Could you check a few things on this model? Use its own coordinates, in mm. A direction names the side the tool comes from. Give positions to 0.01 mm unless a question says otherwise; leave off trailing zeros. Order: outer loops, then holes, each group sorted by start corner. A loop starts at its lowest first (then second) coordinate and runs counter-clockwise, first axis right, second up. Notation, with made-up numbers: (-1.75, 44) -> (23.25, 44) arc R22 cw to (23.25, 60) -> close; hole circle Ø5 at (71.25, -21). An arc over 180 degrees is marked (long way). Use one line per item in the form item = value. Start each with the question number.
from build123d import *

# Parameters (mm, degrees)
BOSS_EXTRUDE13_OUTLINE_W = 40
BOSS_EXTRUDE13_OUTLINE_H = 40
BOSS_EXTRUDE13_OUTLINE_R = 2.5
BOSS_EXTRUDE13_DEPTH     = 5
SKETCH3_R                = 12
BOSS_EXTRUDE17_DEPTH     = 30
FILLET2_R                = 1
FILLET3_R                = 5
FILLET4_R                = 1
SKETCH6_R                = 16
BOSS_EXTRUDE18_DEPTH     = 6
SKETCH5_R                = 6.5
CUT_EXTRUDE2_DEPTH       = 55


# Read off the part's stored shape, not the designer's step: Boss-Extrude13
with BuildPart() as part:
    # Boss-Extrude13 outline → Boss-Extrude13 (new body)
    with BuildSketch(Plane(origin=(0, 0, 0), x_dir=(1, 0, 0), z_dir=(0, 1, 0))):
        Rectangle(BOSS_EXTRUDE13_OUTLINE_W, BOSS_EXTRUDE13_OUTLINE_H)
        with Locations((-15, -15.102802021)):
            Circle(BOSS_EXTRUDE13_OUTLINE_R, mode=Mode.SUBTRACT)
        with Locations((15.102802021, -15.102802021)):
            Circle(BOSS_EXTRUDE13_OUTLINE_R, mode=Mode.SUBTRACT)
        with Locations((-15, 15)):
            Circle(BOSS_EXTRUDE13_OUTLINE_R, mode=Mode.SUBTRACT)
        with Locations((15.102802021, 15)):
            Circle(BOSS_EXTRUDE13_OUTLINE_R, mode=Mode.SUBTRACT)
    extrude(amount=BOSS_EXTRUDE13_DEPTH)

    # Sketch3 → Boss-Extrude17 (add)
    with BuildSketch(Plane(origin=(0, 5, 0), x_dir=(1, 0, 0), z_dir=(0, 1, 0))):
        with Locations(Location((0, 0, 0), (0, 0, 270))):
            Circle(SKETCH3_R)
    extrude(amount=BOSS_EXTRUDE17_DEPTH)

    # Fillet2
    fillet2_edges = [part.edges().sort_by_distance(p)[0] for p in [
        (20, 5, 0),
        (0, 5, -20),
        (-20, 5, 0),
        (0, 5, 20),
    ]]
    fillet(fillet2_edges, radius=FILLET2_R)

    # Fillet3
    # the kernel refuses this fillet: 5 mm, written as the material it adds along each edge
    with BuildSketch(Plane(origin=(0, 5, 0), x_dir=(0, 0, 1), z_dir=(-1, 0, 0))) as fillet3_piece_1:
        with BuildLine():
            CenterArc((12 + FILLET3_R, FILLET3_R), FILLET3_R, 180, 90)
            Line((12, FILLET3_R), (12, 0))
            Line((12, 0), (12 + FILLET3_R, 0))
        make_face()
    revolve(axis=Axis((0, 5, 0), (0, 1, 0)))
    # the kernel refuses this fillet: 5 mm, written as the material it takes off along each edge
    with BuildSketch(Plane(origin=(-15, 5, -15), x_dir=(0, 0, -1), z_dir=(1, 0, 0))) as fillet3_2_piece_1:
        with BuildLine():
            CenterArc((4, -1), 1, 0, 90)
            Line((5, -1), (5, 0))
            Line((5, 0), (4, 0))
        make_face()
    revolve(axis=Axis((-15, 5, -15), (0, 1, 0)), revolution_arc=90, mode=Mode.SUBTRACT)
    with BuildSketch(Plane(origin=(15, 5, -15), x_dir=(1, 0, 0), z_dir=(0, 0, 1))) as fillet3_2_piece_2:
        with BuildLine():
            CenterArc((4, -1), 1, 0, 90)
            Line((5, -1), (5, 0))
            Line((5, 0), (4, 0))
        make_face()
    revolve(axis=Axis((15, 5, -15), (0, 1, 0)), revolution_arc=90, mode=Mode.SUBTRACT)
    with BuildSketch(Plane(origin=(-15, 5, 15), x_dir=(-1, 0, 0), z_dir=(0, 0, -1))) as fillet3_2_piece_3:
        with BuildLine():
            CenterArc((4, -1), 1, 0, 90)
            Line((5, -1), (5, 0))
            Line((5, 0), (4, 0))
        make_face()
    revolve(axis=Axis((-15, 5, 15), (0, 1, 0)), revolution_arc=90, mode=Mode.SUBTRACT)
    with BuildSketch(Plane(origin=(15, 5, 15), x_dir=(0, 0, 1), z_dir=(-1, 0, 0))) as fillet3_2_piece_4:
        with BuildLine():
            CenterArc((4, -1), 1, 0, 90)
            Line((5, -1), (5, 0))
            Line((5, 0), (4, 0))
        make_face()
    revolve(axis=Axis((15, 5, 15), (0, 1, 0)), revolution_arc=90, mode=Mode.SUBTRACT)
    with BuildSketch(Plane(origin=(20, -12.5, 20), x_dir=(-1, 0, 0), z_dir=(0, 1, 0)), Plane(origin=(20, -12.5, -20), x_dir=(0, 0, 1), z_dir=(0, 1, 0))) as fillet3_2_piece_5:
        with BuildLine():
            CenterArc((FILLET3_R, -FILLET3_R), FILLET3_R, 90, 90)
            Line((0, -FILLET3_R), (0, 0))
            Line((0, 0), (FILLET3_R, 0))
        make_face()
    extrude(amount=17.5, mode=Mode.SUBTRACT)
    with BuildSketch(Plane(origin=(-20, -12.5, 20), x_dir=(1, 0, 0), z_dir=(0, 1, 0)), Plane(origin=(-20, -12.5, -20), x_dir=(0, 0, 1), z_dir=(0, 1, 0))) as fillet3_2_piece_6:
        with BuildLine():
            CenterArc((FILLET3_R, FILLET3_R), FILLET3_R, 180, 90)
            Line((0, FILLET3_R), (0, 0))
            Line((0, 0), (FILLET3_R, 0))
        make_face()
    extrude(amount=17.5, mode=Mode.SUBTRACT)

    # Fillet4
    fillet4_edges = [part.edges().sort_by_distance(p)[0] for p in [
        (0, 35, -12),
    ]]
    fillet(fillet4_edges, radius=FILLET4_R)

    # Sketch6 → Boss-Extrude18 (add)
    with BuildSketch(Plane.XZ):
        with Locations(Location((0, 0, 0), (0, 0, 90))):
            Circle(SKETCH6_R)
    extrude(amount=BOSS_EXTRUDE18_DEPTH)

    # Sketch5 → Cut-Extrude2 (cut)
    with BuildSketch(Plane(origin=(0, 35, 0), x_dir=(1, 0, 0), z_dir=(0, 1, 0))):
        with Locations(Location((0, 0, 0), (0, 0, 270))):
            Circle(SKETCH5_R)
    extrude(amount=-CUT_EXTRUDE2_DEPTH, mode=Mode.SUBTRACT)


solid = part.part
(1) We'd pull the mould along X, two halves only. Please class faces 4 (the cylindrical face through (19, 2, -18)), 5 (the cylindrical face through (-19, 2, 18)), 6 (the cylindrical face through (-15.542, 2.465, 17.543)), 7 (the cylindrical face through (3.604, 21.832, 11.446)): pulls with the +X half, pulls with the -X half, needs draft (parallel to the pull), parting line crosses it, or undercut.
(2) Imagine slicing it at D-D (x = 14). Give the number of separate pieces and of enclosed holes in the cut face, plus the area to 3 significant figures.
(3) Imagine slicing it at C-C (y = 23). Write out the boundary of the cut face in (x, z).
(4) Which directions (+Z, -Z, +X, -X, +Y, -Y) give clear straight access to the entire face, cutting with the end or side of a thin tool? Please do faces 1 (the flat face through (-9, 0, -14)), 2 (the flat face through (-17.2, 5, -0.3)), 3 (the flat face through (20, 2, 0)).
(5) I'm going to push flat-ended pins straight in: pin 1 Ø3 at (x, y) = (10, 13.5) entering from -Z; pin 2 Ø5 at (y, z) = (19.5, 4.5) entering from -X; pin 3 Ø2 at (y, z) = (8.5, -2.5) entering from -X. Where does each tip first touch, or does it pass through?
(6) Please list where these lines run through material, in increasing order: probe 1 along Z at (x, y) = (-15, 3.2); probe 2 along Y at (x, z) = (-17.5, 4).
(7) Imagine slicing it at A-A (z = 0). Write out the boundary of the cut face in (x, y), plus the area to 3 significant figures.
(8) Imagine slicing it at B-B (x = 0). Write out the boundary of the cut face in (y, z), plus the area to 3 significant figures.
Calculated:
q1.face_4 = pulls with the +X half
q1.face_5 = pulls with the -X half
q1.face_6 = undercut
q1.face_7 = parting line crosses it
q2.separate_pieces = 3
q2.enclosed_holes = 0
q2.area = 257 mm2
q3.outline = circle Ø24 at (0, 0); hole circle Ø13 at (0, 0)
q4.face_1 = -Y
q4.face_2 = +Y
q4.face_3 = +Z, -Z, +X, +Y, -Y
q5.pin_1 = -8.47
q5.pin_2 = -11.83
q5.pin_3 = -12.45
q6.probe_1 = -20 to -17.5, -12.5 to 12.6, 17.6 to 20
q6.probe_2 = 0 to 5
q7.outline = (-20, 0) -> (-16, 0) -> (-16, -6) -> (-6.5, -6) -> (-6.5, 35) -> (-11, 35) arc R1 ccw to (-12, 34) -> (-12, 10) arc R5 cw to (-17, 5) -> (-19, 5) arc R1 ccw to (-20, 4) -> close; (6.5, -6) -> (16, -6) -> (16, 0) -> (20, 0) -> (20, 4) arc R1 ccw to (19, 5) -> (17, 5) arc R5 cw to (12, 10) -> (12, 34) arc R1 ccw to (11, 35) -> (6.5, 35) -> close
q7.area = 589 mm2
q8.outline = (-6, -16) -> (0, -16) -> (0, -20) -> (4, -20) arc R1 ccw to (5, -19) -> (5, -17) arc R5 cw to (10, -12) -> (34, -12) arc R1 ccw to (35, -11) -> (35, -6.5) -> (-6, -6.5) -> close; (-6, 6.5) -> (35, 6.5) -> (35, 11) arc R1 ccw to (34, 12) -> (10, 12) arc R5 cw to (5, 17) -> (5, 19) arc R1 ccw to (4, 20) -> (0, 20) -> (0, 16) -> (-6, 16) -> close
q8.area = 589 mm2
